Autodesk Inventor part; units mm, degrees
ref_plane "YZ Plane" through (0, 0, 0) normal (1, 0, 0) x (0, 1, 0)
ref_plane "XZ Plane" through (0, 0, 0) normal (0, 1, 0) x (-1, 0, 0)
ref_plane "XY Plane" through (0, 0, 0) normal (0, 0, 1) x (1, 0, 0)
sketch "Skizze2" plane through (0, 0, 0) normal (1, 0, 0) x (0, 1, 0)
  line L0 (0, 0) -> (18.8, 0)
  line L1 (3.3, 18) -> (14.3, 18)
  line L2 (18.8, 31.354) -> (17.3, 31.9)
  line L3 (17.3, 31.9) -> (14.3, 31.9)
  line L4 (14.3, 31.9) -> (14.3, 30.15)
  line L5 (14.3, 30.15) -> (10.8, 30.15)
  line L6 (10.8, 30.15) -> (10.8, 31.9)
  line L7 (10.8, 31.9) -> (7.8, 31.9)
  line L8 (7.8, 31.9) -> (7.8, 35)
  line L9 (7.8, 35) -> (0, 35)
  line L10 (0, 35) -> (0, 31.5)
  line L11 (0, 31.5) -> (2.5, 31.5)
  line L12 (2.5, 31.5) -> (2.5, 25)
  line L13 (2.5, 25) -> (4.8, 25)
  line L14 (4.8, 25) -> (4.8, 21)
  line L15 (4.8, 21) -> (3.3, 21)
  line L16 (3.3, 21) -> (3.3, 18)
  line L17 (18.8, 31.354) -> (18.8, 27.5)
  line L18 (18.8, 27.5) -> (14.3, 27.5)
  line L19 (14.3, 27.5) -> (14.3, 18)
  dimension "d5" = 36
  dimension "d10" = 20
  dimension "d11" = 60.3
  dimension "d12" = 63.8
  dimension "d15" = 3
  dimension "d16" = 1.5
  dimension "d17" = 4
  dimension "d19" = 2.3
  dimension "d20" = 63
  dimension "d26" = 70
  dimension "d28" = 2.5
  dimension "d33" = 11
  dimension "d34" = 1.5
  dimension "d35" = 4.5
  dimension "d36" = 8
  dimension "d37" = 11
  dimension "d53" = 55
  dimension "d54" = 4.5
revolve "Umdrehung1" add sketch "Skizze2" angle 360 about axis through (0, 0, 0) along (0, 1, 0)
fillet "Rundung1" radius 0.3 4 edges at (0, 10.8, -30.15) (0, 14.3, -30.15) (0, 10.8, -31.9) (0, 14.3, -31.9)
sketch "Skizze5" plane through (0, 2.5, 0) normal (0, -1, 0) x (1, 0, 0)
  line L0 (0, 0) -> (35, 0) construction
  circle A0 centre (0, 0) radius 35 construction
  point P0 (28.15, 0)
  point P1 (14.075, 24.3786)
  point P2 (-14.075, 24.3786)
  point P3 (-28.15, 0)
  point P4 (-14.075, -24.3786)
  point P5 (14.075, -24.3786)
  dimension "d58" = 28.15
  dimension "d61" = 360
hole "Bohrung3" at (28.15, 2.5, 0) at (14.075, 2.5, 24.3786) at (-14.075, 2.5, 24.3786) at (-28.15, 2.5, 0) at (-14.075, 2.5, -24.3786) at (14.075, 2.5, -24.3786) direction (0, 1, 0) diameter 2.459 depth 6.5 tip angle 118
sketch "Skizze6" plane through (0, 14.3, 0) normal (0, 1, 0) x (1, 0, 0)
  circle A0 centre (0, 0) radius 22.65
  point P0 (0, 23.65)
  point P1 (20.45, -9.7376)
  point P2 (-20.45, -9.7376)
  dimension "d72" = 45.3
  dimension "d70" = 23.65
  dimension "d71" = 40.9
hole "Bohrung5" at (0, 14.3, -23.65) at (20.45, 14.3, 9.7376) at (-20.45, 14.3, 9.7376) direction (0, -1, 0) diameter 2.5 depth 6 tip angle 118
thread "Gewinde1"
thread "Gewinde2"
thread "Gewinde3"
equation "\"d36\" = d35 + ORing1"
equation "\"ORing1\" = 3.5"
properties part number "Deckel_unten_BFA_35_30_10" material "PVC, hart"
Input: part model. Units: mm. Frame: model coordinates. A direction names the side the tool comes from. Give positions to 0.01 mm unless a question says otherwise; leave off trailing zeros. Return JSON: item names as keys, results as strings.
Item 1: First-contact query: P1, Ø4, axis at x = 5, z = -19.5, coming from the +Y side; P2, Ø25, axis at x = -10.5, z = -12, coming from the -Y side; P3, Ø2, axis at y = 4, z = 13, coming from the -X side. Flat tips, straight axial feed; report the tip coordinate or a pass-through.
Solutions:
{"P1": "y = 14.3", "P2": "y = 2.5", "P3": "x = -32.88"}
Item 2: Ray query, probe 1 along X at (y, z) = (4.35, 0); probe 2 along Z at (x, y) = (-13.5, 9); probe 3 along Y at (x, z) = (10, -16). Return the intervals inside material, ascending.
Solutions:
{"probe 1": "-35 to -29.38, -26.92 to -25, -21 to -18, 18 to 21, 25 to 26.92, 29.38 to 35", "probe 2": "-28.9 to -25.47, -23.29 to -11.91, 11.91 to 23.29, 25.47 to 28.9", "probe 3": "3.3 to 14.3"}
Item 3: Access query for faces 1 (the flat face through (-28, 18.8, 0)), 2 (the flat face through (16, 3.3, -9)), 3 (the cylindrical face through (21.56, 11.26, 10.31)). Directions: +Z, -Z, +X, -X, +Y, -Y. A direction counts if a zero-diameter tool reaches every point of the face in a straight line with its end or side. Return the directions, or none.
Solutions:
{"face 1": "+Z, -Z, +X, -X, +Y", "face 2": "-Y", "face 3": "+Y"}
